from build123d import *

# Parameters (mm, degrees)
ESQUISSE1_W             = 40
ESQUISSE1_H             = 41.3
BOSS_EXTRU_1_DEPTH      = 12.5
BOSS_EXTRU_1_DEPTH_BACK = 12.5
ENL_V_MAT_EXTRU_1_REACH = 27
ENL_V_MAT_EXTRU_2_REACH = 43.3
ESQUISSE3_R             = 1.6
ENL_V_MAT_EXTRU_3_REACH = 43.3
ESQUISSE4_R             = 1.6
CHANFREIN7_SIZE         = 1.8
CONG_4_R                = 2


with BuildPart() as part:
    # Esquisse1 → Boss.-Extru.1 (new body, two sides)
    with BuildSketch(Plane.XY) as boss_extru_1_sk:
        Rectangle(ESQUISSE1_W, ESQUISSE1_H)
    extrude(amount=BOSS_EXTRU_1_DEPTH)
    extrude(boss_extru_1_sk.sketch, amount=-BOSS_EXTRU_1_DEPTH_BACK)

    # Esquisse2 → Enl_v. mat.-Extru.1 (cut, up to next)
    with BuildSketch(Plane.XY.offset(12.5), mode=Mode.PRIVATE) as enl_v_mat_extru_1_sk1:
        with BuildLine():
            Line((-20, 15.65), (-20, -15.65))
            ThreePointArc((-20, -15.65), (-15.594481827, 0), (-20, 15.65))
        make_face()
    enl_v_mat_extru_1_tool1 = extrude(enl_v_mat_extru_1_sk1.sketch, amount=-ENL_V_MAT_EXTRU_1_REACH, mode=Mode.PRIVATE) & part.part
    add(enl_v_mat_extru_1_tool1.solids().sort_by_distance((-18.226209, 0, 12.5))[0], mode=Mode.SUBTRACT)
    # Esquisse2 → Enl_v. mat.-Extru.1 (cut, up to next)
    with BuildSketch(Plane.XY.offset(12.5), mode=Mode.PRIVATE) as enl_v_mat_extru_1_sk2:
        with BuildLine():
            Line((20, 15.65), (20, -15.65))
            ThreePointArc((20, -15.65), (15.594481827, 0), (20, 15.65))
        make_face()
    enl_v_mat_extru_1_tool2 = extrude(enl_v_mat_extru_1_sk2.sketch, amount=-ENL_V_MAT_EXTRU_1_REACH, mode=Mode.PRIVATE) & part.part
    add(enl_v_mat_extru_1_tool2.solids().sort_by_distance((18.226209, 0, 12.5))[0], mode=Mode.SUBTRACT)
    # Esquisse2 → Enl_v. mat.-Extru.1 (cut, up to next)
    with BuildSketch(Plane.XY.offset(12.5), mode=Mode.PRIVATE) as enl_v_mat_extru_1_sk3:
        with BuildLine():
            Line((-14, -15.65), (14, -15.65))
            ThreePointArc((14, -15.65), (11.637851253, -9.491102252), (10.46424155, -3))
            Line((10.46424155, -3), (-10.46424155, -3))
            ThreePointArc((-10.46424155, -3), (-11.637851253, -9.491102252), (-14, -15.65))
        make_face()
    enl_v_mat_extru_1_tool3 = extrude(enl_v_mat_extru_1_sk3.sketch, amount=-ENL_V_MAT_EXTRU_1_REACH, mode=Mode.PRIVATE) & part.part
    add(enl_v_mat_extru_1_tool3.solids().sort_by_distance((0, -9.638348, 12.5))[0], mode=Mode.SUBTRACT)
    # Esquisse2 → Enl_v. mat.-Extru.1 (cut, up to next)
    with BuildSketch(Plane.XY.offset(12.5), mode=Mode.PRIVATE) as enl_v_mat_extru_1_sk4:
        with BuildLine():
            Line((-14, 15.65), (14, 15.65))
            ThreePointArc((14, 15.65), (11.637851253, 9.491102252), (10.46424155, 3))
            Line((10.46424155, 3), (-10.46424155, 3))
            ThreePointArc((-10.46424155, 3), (-11.637851253, 9.491102252), (-14, 15.65))
        make_face()
    enl_v_mat_extru_1_tool4 = extrude(enl_v_mat_extru_1_sk4.sketch, amount=-ENL_V_MAT_EXTRU_1_REACH, mode=Mode.PRIVATE) & part.part
    add(enl_v_mat_extru_1_tool4.solids().sort_by_distance((0, 9.638348, 12.5))[0], mode=Mode.SUBTRACT)

    # Esquisse3 → Enl_v. mat.-Extru.2 (cut, up to next)
    with BuildSketch(Plane(origin=(0, 20.65, 0), x_dir=(1, 0, 0), z_dir=(0, 1, 0)), mode=Mode.PRIVATE) as enl_v_mat_extru_2_sk1:
        with Locations((-9, 0)):
            Circle(ESQUISSE3_R)
    enl_v_mat_extru_2_tool1 = extrude(enl_v_mat_extru_2_sk1.sketch, amount=-ENL_V_MAT_EXTRU_2_REACH, mode=Mode.PRIVATE) & part.part
    add(enl_v_mat_extru_2_tool1.solids().sort_by_distance((-9, 20.65, 0))[0], mode=Mode.SUBTRACT)
    # Esquisse3 → Enl_v. mat.-Extru.2 (cut, up to next)
    with BuildSketch(Plane(origin=(0, 20.65, 0), x_dir=(1, 0, 0), z_dir=(0, 1, 0)), mode=Mode.PRIVATE) as enl_v_mat_extru_2_sk2:
        with Locations((9, 0)):
            Circle(ESQUISSE3_R)
    enl_v_mat_extru_2_tool2 = extrude(enl_v_mat_extru_2_sk2.sketch, amount=-ENL_V_MAT_EXTRU_2_REACH, mode=Mode.PRIVATE) & part.part
    add(enl_v_mat_extru_2_tool2.solids().sort_by_distance((9, 20.65, 0))[0], mode=Mode.SUBTRACT)

    # Esquisse4 → Enl_v. mat.-Extru.3 (cut, up to next)
    with BuildSketch(Plane.XZ.offset(20.65), mode=Mode.PRIVATE) as enl_v_mat_extru_3_sk1:
        with Locations((-9, 0)):
            Circle(ESQUISSE4_R)
    enl_v_mat_extru_3_tool1 = extrude(enl_v_mat_extru_3_sk1.sketch, amount=-ENL_V_MAT_EXTRU_3_REACH, mode=Mode.PRIVATE) & part.part
    add(enl_v_mat_extru_3_tool1.solids().sort_by_distance((-9, -20.65, 0))[0], mode=Mode.SUBTRACT)
    # Esquisse4 → Enl_v. mat.-Extru.3 (cut, up to next)
    with BuildSketch(Plane.XZ.offset(20.65), mode=Mode.PRIVATE) as enl_v_mat_extru_3_sk2:
        with Locations((9, 0)):
            Circle(ESQUISSE4_R)
    enl_v_mat_extru_3_tool2 = extrude(enl_v_mat_extru_3_sk2.sketch, amount=-ENL_V_MAT_EXTRU_3_REACH, mode=Mode.PRIVATE) & part.part
    add(enl_v_mat_extru_3_tool2.solids().sort_by_distance((9, -20.65, 0))[0], mode=Mode.SUBTRACT)

    # Chanfrein7
    chanfrein7_edges = [part.edges().sort_by_distance(p)[0] for p in [
        (-15.594481827, 0, 12.5),
        (-15.594481827, 0, -12.5),
        (0, 15.65, 12.5),
        (0, 3, 12.5),
        (0, 15.65, -12.5),
        (0, 3, -12.5),
        (0, -15.65, 12.5),
        (0, -3, 12.5),
        (0, -15.65, -12.5),
        (0, -3, -12.5),
        (15.594481827, 0, 12.5),
        (15.594481827, 0, -12.5),
    ]]
    chamfer(chanfrein7_edges, length=CHANFREIN7_SIZE)

    # Cong_4
    cong_4_edges = [part.edges().sort_by_distance(p)[0] for p in [
        (10.46424155, -3, 0),
        (-10.46424155, -3, 0),
        (-10.46424155, 3, 0),
        (10.46424155, 3, 0),
    ]]
    fillet(cong_4_edges, radius=CONG_4_R)


solid = part.part
Build history of the part. All positions in model axes, mm. A direction names the side the tool comes from. Give positions to 0.01 mm unless a question says otherwise; leave off trailing zeros. Order: outer loops, then holes, each group sorted by start corner. A loop starts at its lowest first (then second) coordinate and runs counter-clockwise, first axis right, second up. Notation, with made-up numbers: M 83.25,39 L 142.25,39 A9 cw 142.25,43 Z; hole C 53,-11.5 d9. An arc over 180 degrees is marked long. Put each result on its own line as item: value.
Item 1: Slice it at C-C, the plane z = 0. Give the number of separate pieces and of enclosed holes in the cut face, plus the area to 3 significant figures.
From the geometry:
separate pieces: 3
enclosed holes: 0
area: 807 mm2
Item 2: Slice it at A-A, the plane x = 3. Write the cut outline in (y, z), plus the area to 3 significant figures.
From the geometry:
outline: M -20.65,-12.5 L -17.45,-12.5 L -15.65,-10.7 L -15.65,10.7 L -17.45,12.5 L -20.65,12.5 Z; M -3,-10.7 L -1.2,-12.5 L 1.2,-12.5 L 3,-10.7 L 3,10.7 L 1.2,12.5 L -1.2,12.5 L -3,10.7 Z; M 15.65,-10.7 L 17.45,-12.5 L 20.65,-12.5 L 20.65,12.5 L 17.45,12.5 L 15.65,10.7 Z
area: 387 mm2
Item 3: Probe line 1 (X direction, y = 16.7, z = 0); line 2 (Y direction, x = -6.5, z = -6.75); line 3 (Z direction, x = 9, y = 19). List the from-to ranges inside material, lowest first. Write a range as [from, to].
From the geometry:
line 1: x = [-20, -10.6], [-7.4, 7.4], [10.6, 20]
line 2: y = [-20.65, -15.65], [-3, 3], [15.65, 20.65]
line 3: z = [-12.5, -1.6], [1.6, 12.5]
Item 4: Flat gauge pins, fed straight in: pin 1 Ø3 at (y, z) = (-13.5, 2.5) entering from +X; pin 2 Ø2.5 at (x, z) = (9, 0) entering from -Y; pin 3 Ø3.5 at (x, z) = (9, 0) entering from -Y; pin 4 Ø5 at (y, z) = (10.5, -7.5) entering from +X. Where does each tip first touch, or does it go through?
From the geometry:
pin 1: stops at x = 19.61
pin 2: stops at y = -3.77
pin 3: stops at y = -20.65
pin 4: stops at x = 18.56
Item 5: Slice it at B-B, the plane z = -2.75. Write the cut outline in (x, y).
From the geometry:
outline: M -20,-20.65 L 20,-20.65 L 20,-15.65 A30 cw 20,15.65 L 20,20.65 L -20,20.65 L -20,15.65 A30 cw -20,-15.65 Z; hole M -14,-15.65 L 14,-15.65 A35.26 cw 10.66,-4.73 A2 ccw 8.67,-3 L -8.67,-3 A2 ccw -10.66,-4.73 A35.26 cw Z; hole M -14,15.65 A35.26 cw -10.66,4.73 A2 ccw -8.67,3 L 8.67,3 A2 ccw 10.66,4.73 A35.26 cw 14,15.65 Z
Item 6: Two-plate mould, pull along Y, no slides. Class faces 4 (the flat face through (20, -18, 0)), 5 (the cylindrical face through (-9.974, 3.481, -0.15)): +Y half, -Y half, draft (parallel to the pull), parting line (faces both ways), or undercut.
From the geometry:
face 4: draft
face 5: undercut
Item 7: 3-axis set-ups, long thin cutter, end or side, ignore diameter. For faces 1 (the flat face through (0, -3, 0)), 2 (the flat face through (-0.21, -16.54, 11.59)), 3 (the flat face through (0.21, 16.54, -11.59)): which of +Z, -Z, +X, -X, +Y, -Y reach the whole face in a straight line?
From the geometry:
face 1: +Z, -Z
face 2: +Z
face 3: -Z
Item 8: Slice it at D-D, the plane x = 8. Write the cut outline in (y, z).
From the geometry:
outline: M -20.65,-12.5 L -17.45,-12.5 L -15.65,-10.7 L -15.65,-1.25 L -20.65,-1.25 Z; M -20.65,1.25 L -15.65,1.25 L -15.65,10.7 L -17.45,12.5 L -20.65,12.5 Z; M -3,-10.7 L -1.2,-12.5 L 1.2,-12.5 L 3,-10.7 L 3,10.7 L 1.2,12.5 L -1.2,12.5 L -3,10.7 Z; M 15.65,-10.7 L 17.45,-12.5 L 20.65,-12.5 L 20.65,-1.25 L 15.65,-1.25 Z; M 15.65,1.25 L 20.65,1.25 L 20.65,12.5 L 17.45,12.5 L 15.65,10.7 Z
